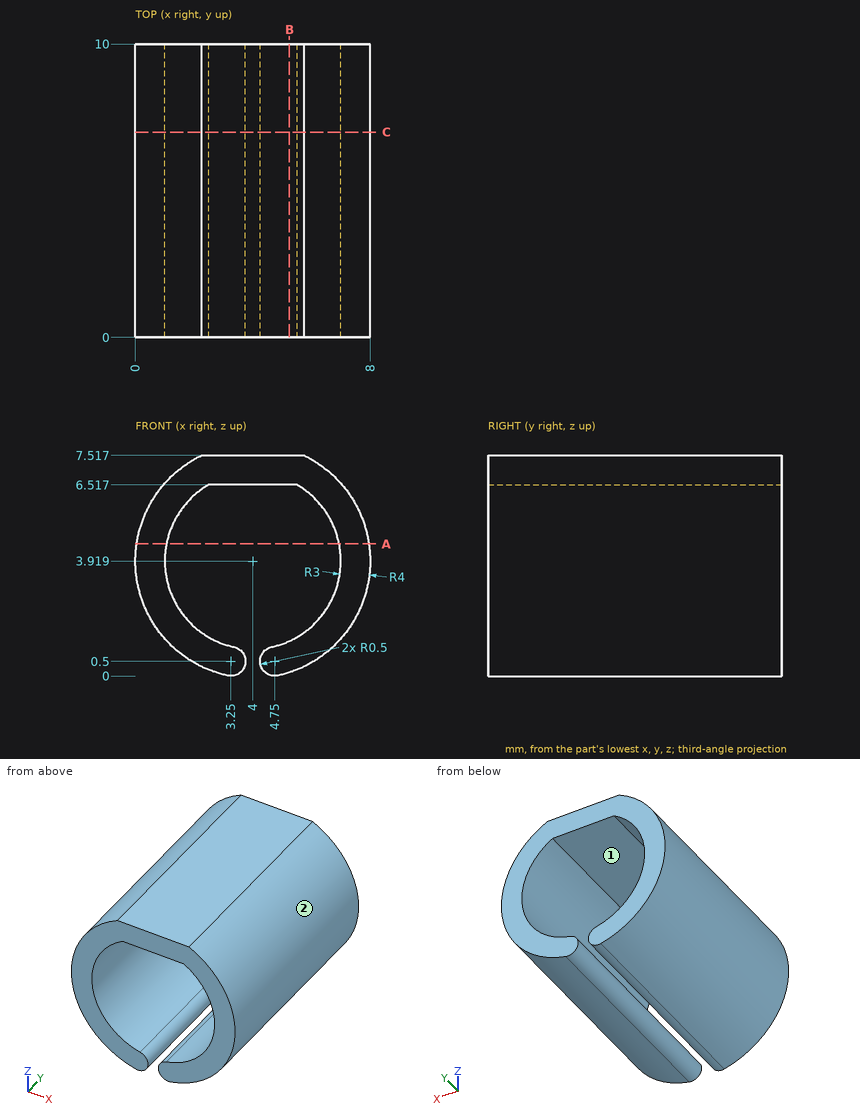
Part print with two shaded views. Sizes in mm from the minimum x, y, z corner. A direction names the side the tool comes from. Round coordinates to 2 decimals unless told otherwise and drop trailing zeros. Order: outer loops, then holes, each group sorted by start corner. A loop starts at its lowest first (then second) coordinate and runs counter-clockwise, first axis right, second up. Notation, with made-up numbers: M 71,16 L 99,16 A6 ccw 99,23 Z; hole C 54.5,74.5 d1. An arc over 180 degrees is marked long. Answer in a Markdown table with one row per item. Add a question column.
Q1. Cut at C-C on y = 7. Give the cut face in (x, z).
Q2. Wall check: L1, parallel to Z at x = 4, y = 9; L2, parallel to X at y = 3, z = 6.25; L3, parallel to Z at x = 4.75, y = 4. Give the ranges that are in metal, low to high. Write a range as from..to.
Q3. Cut at B-B on x = 5.25. Give the cut face in (y, z).
Q4. Cut at A-A on z = 4.5. Give the cut face in (x, y), and give its area (3 significant figures).
Q5. Pin check, flat tips, straight feed: pin 1 (2 mm diameter, centred on x = 6, y = 2, fed in from -Z); pin 2 (3 mm diameter, centred on x = 4, z = 4, fed in from -Y). Stop position of each tip, or through.
Q6. 3-axis set-ups, long thin cutter, end or side, ignore diameter. For the marked faces 1 and 2: which of +Z, -Z, +X, -X, +Y, -Y reach the whole face in a straight line?
Established:
| question | item | result |
|---|---|---|
| 1 | outline | M 2.25,7.52 A4 ccw 3.14,0.01 A0.5 ccw 3.36,0.99 A3 cw 2.5,6.52 L 5.5,6.52 A3 cw 4.64,0.99 A0.5 ccw 4.86,0.01 A4 ccw 5.75,7.52 Z |
| 2 | L1 | z = 6.52..7.52 |
| 2 | L2 | x = 0.75..2.11, 5.89..7.25 |
| 2 | L3 | z = 0..1.01, 6.52..7.52 |
| 3 | outline | M 0,0.12 L 10,0.12 L 10,1.19 L 0,1.19 Z; M 0,6.52 L 10,6.52 L 10,7.52 L 0,7.52 Z |
| 4 | outline | M 0.04,0 L 1.06,0 L 1.06,10 L 0.04,10 Z; M 6.94,0 L 7.96,0 L 7.96,10 L 6.94,10 Z |
| 4 | area | 20.3 mm2 |
| 5 | pin 1 | stops at z = 0.05 |
| 5 | pin 2 | passes through |
| 6 | face 1 | +Y, -Y |
| 6 | face 2 | +X, +Y, -Y |
